from build123d import *

# Parameters (mm, degrees)
SKETCH1_R           = 3.81
SKETCH1_R_2         = 1.27
SKETCH1_R_3         = 3.175
BOSS_EXTRUDE1_DEPTH = 5.9944
FILLET1_R           = 12.7
FILLET2_R           = 12.7


with BuildPart() as part:
    # Sketch1 → Boss-Extrude1 (new body)
    with BuildSketch(Plane.XY):
        with BuildLine():
            Line((-46.655107065, 20.09828313), (0, -19.05))
            Line((0, -19.05), (46.655107065, 20.09828313))
            ThreePointArc((46.655107065, 20.09828313), (0, 50.8), (-46.655107065, 20.09828313))
        make_face()
        with Locations((-10.682756087, 39.86858848)):
            Circle(SKETCH1_R, mode=Mode.SUBTRACT)
        with Locations((10.682756087, 39.86858848)):
            Circle(SKETCH1_R, mode=Mode.SUBTRACT)
        with Locations((-14.8174226, 14.8174226)):
            Circle(SKETCH1_R_2, mode=Mode.SUBTRACT)
        with Locations((-8.980256121, 8.980256121)):
            Circle(SKETCH1_R_2, mode=Mode.SUBTRACT)
        with Locations((8.980256121, 8.980256121)):
            Circle(SKETCH1_R_2, mode=Mode.SUBTRACT)
        with Locations((14.8174226, 14.8174226)):
            Circle(SKETCH1_R_2, mode=Mode.SUBTRACT)
        Circle(SKETCH1_R_3, mode=Mode.SUBTRACT)
    extrude(amount=BOSS_EXTRUDE1_DEPTH)

    # Fillet1
    fillet1_edges = [part.edges().sort_by_distance(p)[0] for p in [
        (46.655107065, 20.09828313, 2.9972),
        (-46.655107065, 20.09828313, 2.9972),
    ]]
    fillet(fillet1_edges, radius=FILLET1_R)

    # Fillet2
    fillet2_edges = [part.edges().sort_by_distance(p)[0] for p in [
        (0, -19.05, 2.9972),
    ]]
    fillet(fillet2_edges, radius=FILLET2_R)


solid = part.part
The listing builds one solid part. Answer for the finished solid, in the listing's coordinates (mm). Give positions to 0.01 mm unless a question says otherwise; leave off trailing zeros. Write each loop counter-clockwise with the first axis right and the second up, starting at its lowest first coordinate (ties: lowest second). Pieces come first, ordered by that corner, then holes. Notation, with made-up numbers: (29.25, 13.5) -> (86.25, 13.5) arc R26 ccw to (86.25, 35.5) -> close; hole circle Ø3 at (-26, 16). An arc over 180 degrees is marked (long way). One line per question, with ' | ' between items. Start each with the question number.
1. Section D-D (y = -7) is taken. Determine the outline of the cut face in (x, z).
2. Section A-A (x = 0) is taken. Determine the outline of the cut face in (y, z) (3 decimals), plus the area to 3 significant figures.
3. Section B-B (z = 4) is taken. State how many separate pieces and enclosed holes the cut face has, plus the area to 3 significant figures.
4. Section C-C (y = 0) is taken. Determine the outline of the cut face in (x, z) (3 decimals), plus the area to 3 significant figures.
5. Given pin 1 Ø1.5 at (x, z) = (-21, 3) entering from +Y, flat-ended and moving along its own axis, determine where the tip first touches the part or whether it passes through.
6. Find the intervals of material crossed by probe 1 along X at (y, z) = (38.5, 2.1); probe 2 along X at (y, z) = (37, 3.65); probe 3 along Y at (x, z) = (9, 3.8), in increasing order.
7. For a pull along X with two mould halves and no side action, classify faces 1 (the cylindrical face through (-0.12, -15.17, 3.04)), 2 (the cylindrical face through (-14.49, 40.04, 2.96)), 3 (the flat face through (-1, 18, 5.994)) as pulls with the +X half, pulls with the -X half, needs draft (parallel to the pull), parting line crosses it, or undercut.
Response values:
1) outline: (-14.36, 0) -> (14.36, 0) -> (14.36, 5.99) -> (-14.36, 5.99) -> close
2) outline: (-15.171, 0) -> (-3.175, 0) -> (-3.175, 5.994) -> (-15.171, 5.994) -> close; (3.175, 0) -> (50.8, 0) -> (50.8, 5.994) -> (3.175, 5.994) -> close | area: 357 mm2
3) separate pieces: 1 | enclosed holes: 7 | area: 3,680 mm2
4) outline: (-22.703, 0) -> (-3.175, 0) -> (-3.175, 5.994) -> (-22.703, 5.994) -> close; (3.175, 0) -> (22.703, 0) -> (22.703, 5.994) -> (3.175, 5.994) -> close | area: 234 mm2
5) pin 1: y = 46.59
6) probe 1: -33.14 to -14.24, -7.13 to 7.13, 14.24 to 33.14 | probe 2: -34.81 to -13.19, -8.18 to 8.18, 13.19 to 34.81 | probe 3: -11.5 to 7.71, 10.25 to 36.45, 43.29 to 50
7) face 1: parting line crosses it | face 2: undercut | face 3: needs draft
